Part model, mm, in its own coordinate system. Round coordinates to 2 decimals unless told otherwise and drop trailing zeros. Write each loop counter-clockwise with the first axis right and the second up, starting at its lowest first coordinate (ties: lowest second). Pieces come first, ordered by that corner, then holes.
1) Flat gauge pins, fed straight in: pin 1 (2.5 mm diameter, centred on x = 10.61, y = -10.61, fed in from +Z); pin 2 (3 mm diameter, centred on x = 15.5, z = 2.5, fed in from -Y); pin 3 (1.5 mm diameter, centred on y = -12, z = 0.5, fed in from +X); pin 4 (3 mm diameter, centred on x = 2.5, z = 1.5, fed in from -Y). Where does each tip first touch, or does it go through?
2) Saw through at C-C on y = 15. Write the cut outline in (x, z), and give its area (3 significant figures).
3) Saw through at A-A on y = 0. Write the cut outline in (x, z).
4) Saw through at D-D on z = 4. Count the separate pieces of the cut face and the enclosed holes in it, and give its area (3 significant figures).
5) Saw through at B-B on x = -15.5. Write the cut outline in (y, z).
6) Drill centre lines: L1, parallel to Y at x = 0, z = 5.25; L2, parallel to Y at x = 1, z = 3.5; L3, parallel to X at y = 0.5, z = 4.25. Where is each one in solid material? Low to high.
7) Pull direction X, two halves, no side cores. Call faces 1 (the cylindrical face through (-1.72, -7.73, 3.25)), 2 (the flat face through (9, 0, 0)), 3 (the cylindrical face through (-4.353, -19.603, 3.254)): +X half, -X half, draft (parallel to the pull), parting line (faces both ways), or undercut.
```python
from build123d import *

# Parameters (mm, degrees)
SKETCH1_R           = 20
SKETCH1_R_2         = 8
SKETCH1_R_3         = 1.75
SKETCH1_R_4         = 1.5
BOSS_EXTRUDE1_DEPTH = 6.6
MOVE_FACE1_BY       = 0.08
MOVE_FACE1_2_BY     = 0.08


with BuildPart() as part:
    # Sketch1 → Boss-Extrude1 (new body)
    with BuildSketch(Plane.XY):
        Circle(SKETCH1_R)
        Circle(SKETCH1_R_2, mode=Mode.SUBTRACT)
        with Locations((0, 15)):
            Circle(SKETCH1_R_3, mode=Mode.SUBTRACT)
        with Locations((10.606601718, 10.606601718)):
            Circle(SKETCH1_R_4, mode=Mode.SUBTRACT)
        with Locations((15, 0)):
            Circle(SKETCH1_R_3, mode=Mode.SUBTRACT)
        with Locations((10.606601718, -10.606601718)):
            Circle(SKETCH1_R_4, mode=Mode.SUBTRACT)
        with Locations((0, -15)):
            Circle(SKETCH1_R_3, mode=Mode.SUBTRACT)
        with Locations((-10.606601718, -10.606601718)):
            Circle(SKETCH1_R_4, mode=Mode.SUBTRACT)
        with Locations((-15, 0)):
            Circle(SKETCH1_R_3, mode=Mode.SUBTRACT)
        with Locations((-10.606601718, 10.606601718)):
            Circle(SKETCH1_R_4, mode=Mode.SUBTRACT)
    extrude(amount=BOSS_EXTRUDE1_DEPTH)

    # Move Face1: a curved face moved outward by 0.08
    add(Solid.thicken(part.faces().sort_by_distance((-8, 0, 3.3))[0], MOVE_FACE1_BY))

    # Move Face1 2: a curved face moved outward by 0.08
    add(Solid.thicken(part.faces().sort_by_distance((-20, 0, 3.3))[0], MOVE_FACE1_2_BY))


solid = part.part
```
Completed:
1. pin 1: passes through
1. pin 2: stops at y = -14.39
1. pin 3: stops at x = 16.63
1. pin 4: stops at y = -20.06
2. outline: (-13.35, 0) - (-1.75, 0) - (-1.75, 6.6) - (-13.35, 6.6) - close; (1.75, 0) - (13.35, 0) - (13.35, 6.6) - (1.75, 6.6) - close
2. area: 153 mm2
3. outline: (-20.08, 0) - (-16.75, 0) - (-16.75, 6.6) - (-20.08, 6.6) - close; (-13.25, 0) - (-7.92, 0) - (-7.92, 6.6) - (-13.25, 6.6) - close; (7.92, 0) - (13.25, 0) - (13.25, 6.6) - (7.92, 6.6) - close; (16.75, 0) - (20.08, 0) - (20.08, 6.6) - (16.75, 6.6) - close
4. separate pieces: 1
4. enclosed holes: 9
4. area: 1,000 mm2
5. outline: (-12.77, 0) - (-1.68, 0) - (-1.68, 6.6) - (-12.77, 6.6) - close; (1.68, 0) - (12.77, 0) - (12.77, 6.6) - (1.68, 6.6) - close
6. L1: y = -20.08 to -16.75, -13.25 to -7.92, 7.92 to 13.25, 16.75 to 20.08
6. L2: y = -20.06 to -16.44, -13.56 to -7.86, 7.86 to 13.56, 16.44 to 20.06
6. L3: x = -20.07 to -16.68, -13.32 to -7.9, 7.9 to 13.32, 16.68 to 20.07
7. face 1: undercut
7. face 2: draft
7. face 3: parting line
